Could you check a few things on this model? Use its own coordinates, in mm. Give positions to 0.01 mm unless a question says otherwise; leave off trailing zeros. Write each loop counter-clockwise with the first axis right and the second up, starting at its lowest first coordinate (ties: lowest second). Pieces come first, ordered by that corner, then holes. Notation, with made-up numbers: (52.5, -31) - (98.5, -31) arc R30 cw to (98.5, -7) - close; hole circle Ø8 at (11, 47). An arc over 180 degrees is marked (long way). Answer in a Markdown table with one row per item.
from build123d import *

# Parameters (mm, degrees)
F0_W     = 25.4
F0_H     = 25.4
F1_DEPTH = 25.4
F4_DEPTH = 25.4
F5_DEPTH = 25.4


with BuildPart() as f1:
    # F0 (on Front) → F1 (new body)
    with BuildSketch(Plane.XZ):
        with Locations((-22.479386, 17.278457)):
            Rectangle(F0_W, F0_H)
    extrude(amount=F1_DEPTH)

    # F3 (on face) → F4 (cut)
    with BuildSketch(Plane(origin=(-35.179386, 0, 0), x_dir=(0, -1, 0), z_dir=(-1, 0, 0))):
        Polygon((25.4, 29.978457), (12.7, 29.978457), (25.4, 17.278457), align=None)
        Polygon((0, 17.278457), (12.7, 29.978457), (0, 29.978457), align=None)
        Polygon((12.7, 4.578457), (0, 17.278457), (0, 4.578457), align=None)
        Polygon((25.4, 4.578457), (25.4, 17.278457), (12.7, 4.578457), align=None)
    extrude(amount=-F4_DEPTH, mode=Mode.SUBTRACT)

    # F2 (on face) → F5 (cut)
    with BuildSketch(Plane.XZ.offset(25.4)):
        Polygon((-9.779386, 29.978457), (-22.479386, 29.978457), (-9.779386, 17.278457), align=None)
        Polygon((-9.779386, 4.578457), (-9.779386, 17.278457), (-22.479386, 4.578457), align=None)
        Polygon((-22.479386, 4.578457), (-35.179386, 17.278457), (-35.179386, 4.578457), align=None)
        Polygon((-35.179386, 17.278457), (-22.479386, 29.978457), (-35.179386, 29.978457), align=None)
    extrude(amount=-F5_DEPTH, mode=Mode.SUBTRACT)


solid = f1.part
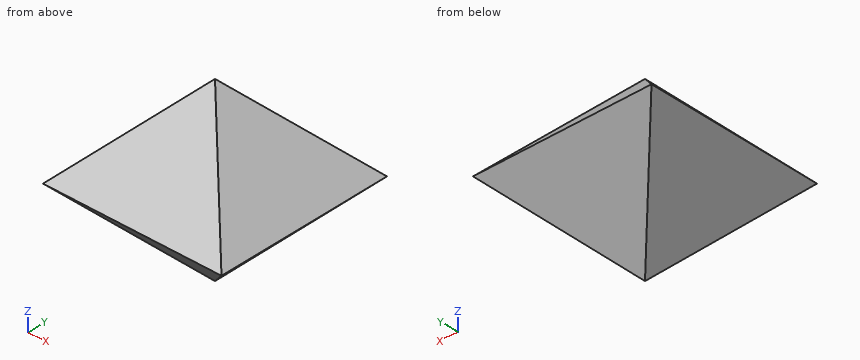
1) If I drill on line 1 (X direction, y = -15.5, z = 9.5); line 2 (Y direction, x = -21.75, z = 24.75); line 3 (X direction, y = -17, z = 20), over which ranges is the centre line in solid material (lowest first)?
Check values:
| item | result |
|---|---|
| line 1 | x = -27.4 to -17.56 |
| line 2 | y = -17.93 to -7.47 |
| line 3 | x = -32.46 to -12.5 |
2) Will these pins go through, and if not, where does the flat tip stop? P1, Ø8, axis at x = -29.5, y = -18.5, coming from the -Z side; P2, Ø1, axis at y = -20.5, z = 16, coming from the -X side; P3, Ø1, axis at x = -32, y = -4.5, coming from the -Z side; P4, Ø1, axis at x = -31.5, z = 17.5, coming from the +Y side.
Check values:
| item | result |
|---|---|
| P1 | stops at z = 8.23 |
| P2 | stops at x = -34.4 |
| P3 | stops at z = 13.6 |
| P4 | stops at y = 0 |
3) Imagine slicing it at A-A (x = -17.5). List the corners of the cut face in (y, z) for me.
Check values:
| item | result |
|---|---|
| outline | (-25.4, 17.28) - (-17.68, 9.56) - (-7.72, 9.56) - (0, 17.28) - (-7.72, 25) - (-17.68, 25) - close |
4) Imagine slicing it at D-D (z = 16.75). List the corners of the cut face in (x, y) for me, then the cut area to 3 significant figures.
Check values:
| item | result |
|---|---|
| outline | (-34.65, -24.87) - (-10.31, -24.87) - (-10.31, -0.53) - (-34.65, -0.53) - close |
| area | 593 mm2 |
5) Imagine slicing it at C-C (z = 23.75). List the corners of the cut face in (x, y) for me.
Check values:
| item | result |
|---|---|
| outline | (-28.71, -18.93) - (-16.25, -18.93) - (-16.25, -6.47) - (-28.71, -6.47) - close |
6) Imagine slicing it at B-B (y = -24). List the corners of the cut face in (x, z) for me, then the cut area to 3 significant figures.
Check values:
| item | result |
|---|---|
| outline | (-35.18, 17.28) - (-33.78, 15.88) - (-11.18, 15.88) - (-9.78, 17.28) - (-11.18, 18.68) - (-33.78, 18.68) - close |
| area | 67.2 mm2 |
